from build123d import *

# Parameters (mm, degrees)
EXTRUDE_1_OUTLINE_W     = 2
EXTRUDE_1_OUTLINE_H     = 2
EXTRUDE_START           = -5
EXTRUDE_1_2_OUTLINE_R   = 4.25
EXTRUDE_1_2_OUTLINE_R_2 = 12
EXTRUDE_1_2_DEPTH       = 10
SKETCH_2_W              = 80
SKETCH_2_H              = 71
EXTRUDE_2_DEPTH         = 10
HOLE_START              = -6
HOLE_WIZARD_4_DEPTH     = 6.7
HOLE_START_2            = 0.7
HOLE_WIZARD_4_2_DEPTH   = 5.3
SKETCH_7_R              = 18
CUT_EXTRUDE_1_DEPTH     = 10
FILLET_2_R              = 5
FILLET_3_R              = 5
SKETCH_8_W              = 52.674698886
SKETCH_8_H              = 88.999999996
EXTRUDE_3_DEPTH         = 10
SKETCH_9_W              = 90.000000011
SKETCH_9_H              = 126.81088124
CUT_EXTRUDE_2_DEPTH     = 10
FILLET_4_R              = 10
FILLET_6_R              = 5


with BuildPart() as part:
    # 凸台-拉伸1: read off the stored shape, not the designer's step
    # 凸台-拉伸1 outline → 凸台-拉伸1 (revolve)
    with BuildSketch(Plane(origin=(0, -22.5, -28.5), x_dir=(0, 1, 0), z_dir=(0, 0, -1))):
        with Locations((11, -4)):
            Rectangle(EXTRUDE_1_OUTLINE_W, EXTRUDE_1_OUTLINE_H)
    revolve(axis=Axis((0, -22.5, -28.5), (1, 0, 0)))

    # Extrude 1 2 outline → Extrude 1 2 (add)
    with BuildSketch(Plane.YZ.offset(EXTRUDE_START)):
        with BuildLine():
            Line((114.999999996, 0), (-40, 0))
            ThreePointArc((-40, 0), (-43.535533906, -1.464466094), (-45, -5))
            Line((-45, -5), (-45, -148))
            Line((-45, -148), (-40, -153))
            Line((-40, -153), (-5, -153))
            Line((-5, -153), (1.7e-08, -147.999999983))
            Line((1.7e-08, -147.999999983), (0, -100))
            ThreePointArc((0, -100), (2.928932188, -92.928932188), (10, -90))
            Line((10, -90), (114.999999996, -90))
            Line((114.999999996, -90), (114.999999996, 0))
        make_face()
        with Locations((-22.5, -130.5)):
            Circle(EXTRUDE_1_2_OUTLINE_R, mode=Mode.SUBTRACT)
        with Locations((-22.5, -85.5)):
            Circle(EXTRUDE_1_2_OUTLINE_R, mode=Mode.SUBTRACT)
        with Locations((-22.5, -28.5)):
            Circle(EXTRUDE_1_2_OUTLINE_R_2, mode=Mode.SUBTRACT)
    extrude(amount=EXTRUDE_1_2_DEPTH)

    # Extrude 1 3 outline → Extrude 1 3 (revolve, cut)
    with BuildSketch(Plane(origin=(0, -22.5, -28.5), x_dir=(0, 1, 0), z_dir=(0, 0, -1))):
        Polygon((12, 5), (12, 4.5), (12.5, 5), align=None)
    revolve(axis=Axis((0, -22.5, -28.5), (1, 0, 0)), mode=Mode.SUBTRACT)

    # 草图2 → 凸台-拉伸2 (add)
    with BuildSketch(Plane.ZY.offset(5)):
        with Locations((40, 79.499999996)):
            Rectangle(SKETCH_2_W, SKETCH_2_H)
    extrude(amount=-EXTRUDE_2_DEPTH)

    # 打孔尺寸(%根据)内六角圆柱头螺钉的类型4: read off the stored shape, not the designer's step
    # 打孔尺寸(%根据)内六角圆柱头螺钉的类型4 outline → 打孔尺寸(%根据)内六角圆柱头螺钉的类型4 (cut)
    with BuildSketch(Plane.YZ.offset(HOLE_START)):
        with BuildLine():
            ThreePointArc((45.508621967, -3.732756057), (50.508621967, -8.732756057), (55.508621967, -3.732756057))
            Line((55.508621967, -3.732756057), (55.508621967, 15.767243943))
            ThreePointArc((55.508621967, 15.767243943), (50.508621967, 20.767243943), (45.508621967, 15.767243943))
            Line((45.508621967, 15.767243943), (45.508621967, -3.732756057))
        make_face()
        with BuildLine():
            ThreePointArc((55.508621967, 73.75), (50.508621967, 78.75), (45.508621967, 73.75))
            Line((45.508621967, 73.75), (45.508621967, 54.25))
            ThreePointArc((45.508621967, 54.25), (50.508621967, 49.25), (55.508621967, 54.25))
            Line((55.508621967, 54.25), (55.508621967, 73.75))
        make_face()
        with BuildLine():
            ThreePointArc((103.491378024, 54.25), (108.491378024, 49.25), (113.491378024, 54.25))
            Line((113.491378024, 54.25), (113.491378024, 73.75))
            ThreePointArc((113.491378024, 73.75), (108.491378024, 78.75), (103.491378024, 73.75))
            Line((103.491378024, 73.75), (103.491378024, 54.25))
        make_face()
        with BuildLine():
            ThreePointArc((113.491378024, 15.767243943), (108.491378024, 20.767243943), (103.491378024, 15.767243943))
            Line((103.491378024, 15.767243943), (103.491378024, -3.732756057))
            ThreePointArc((103.491378024, -3.732756057), (108.491378024, -8.732756057), (113.491378024, -3.732756057))
            Line((113.491378024, -3.732756057), (113.491378024, 15.767243943))
        make_face()
    extrude(amount=HOLE_WIZARD_4_DEPTH, mode=Mode.SUBTRACT)

    # Hole Wizard 4 2 outline → Hole Wizard 4 2 (cut)
    with BuildSketch(Plane.YZ.offset(HOLE_START_2)):
        with BuildLine():
            ThreePointArc((47.758621967, -3.732756057), (50.508621967, -6.482756057), (53.258621967, -3.732756057))
            Line((53.258621967, -3.732756057), (53.258621967, 15.767243943))
            ThreePointArc((53.258621967, 15.767243943), (50.508621967, 18.517243943), (47.758621967, 15.767243943))
            Line((47.758621967, 15.767243943), (47.758621967, -3.732756057))
        make_face()
        with BuildLine():
            ThreePointArc((53.258621967, 73.75), (50.508621967, 76.5), (47.758621967, 73.75))
            Line((47.758621967, 73.75), (47.758621967, 54.25))
            ThreePointArc((47.758621967, 54.25), (50.508621967, 51.5), (53.258621967, 54.25))
            Line((53.258621967, 54.25), (53.258621967, 73.75))
        make_face()
        with BuildLine():
            ThreePointArc((105.741378024, 54.25), (108.491378024, 51.5), (111.241378024, 54.25))
            Line((111.241378024, 54.25), (111.241378024, 73.75))
            ThreePointArc((111.241378024, 73.75), (108.491378024, 76.5), (105.741378024, 73.75))
            Line((105.741378024, 73.75), (105.741378024, 54.25))
        make_face()
        with BuildLine():
            ThreePointArc((111.241378024, 15.767243943), (108.491378024, 18.517243943), (105.741378024, 15.767243943))
            Line((105.741378024, 15.767243943), (105.741378024, -3.732756057))
            ThreePointArc((105.741378024, -3.732756057), (108.491378024, -6.482756057), (111.241378024, -3.732756057))
            Line((111.241378024, -3.732756057), (111.241378024, 15.767243943))
        make_face()
    extrude(amount=HOLE_WIZARD_4_2_DEPTH, mode=Mode.SUBTRACT)

    # 草图7 → 切除-拉伸1 (cut)
    with BuildSketch(Plane.ZY.offset(5)):
        with Locations((35.008621971, 64.999999996)):
            Circle(SKETCH_7_R)
    extrude(amount=-CUT_EXTRUDE_1_DEPTH, mode=Mode.SUBTRACT)

    # 圆角2
    fillet_2_edges = [part.edges().sort_by_distance(p)[0] for p in [
        (0, 114.999999996, -90),
        (0, 114.999999996, 80),
        (0, 43.999999996, 80),
    ]]
    fillet(fillet_2_edges, radius=FILLET_2_R)

    # 圆角3
    fillet_3_edges = [part.edges().sort_by_distance(p)[0] for p in [
        (0, 43.999999996, 0),
    ]]
    fillet(fillet_3_edges, radius=FILLET_3_R)

    # 草图8 → 凸台-拉伸3 (add)
    with BuildSketch(Plane.ZY.offset(5)):
        with Locations((18.662650557, -0.500000002)):
            Rectangle(SKETCH_8_W, SKETCH_8_H)
    extrude(amount=-EXTRUDE_3_DEPTH)

    # 草图9 → 切除-拉伸2 (cut)
    with BuildSketch(Plane.ZY.offset(5)):
        with Locations((-54.999999997, 63.40544062)):
            Rectangle(SKETCH_9_W, SKETCH_9_H)
    extrude(amount=-CUT_EXTRUDE_2_DEPTH, mode=Mode.SUBTRACT)

    # 圆角4
    fillet_4_edges = [part.edges().sort_by_distance(p)[0] for p in [
        (0, 43.999999996, 45),
        (0, 0, -9.999999991),
    ]]
    fillet(fillet_4_edges, radius=FILLET_4_R)

    # 圆角6
    fillet_6_edges = [part.edges().sort_by_distance(p)[0] for p in [
        (0, -45, 45),
        (0, 114.999999996, -9.999999991),
    ]]
    fillet(fillet_6_edges, radius=FILLET_6_R)


solid = part.part
Can you work these out from the model? Positions are in its coordinate system, mm. A direction names the side the tool comes from. Coordinates: 2 decimals unless noted, no trailing zeros. Write each loop counter-clockwise with the first axis right and the second up, starting at its lowest first coordinate (ties: lowest second). Pieces come first, ordered by that corner, then holes. Notation, with made-up numbers: (56, -39.75) - (67, -39.75) arc R8 ccw to (67, -34.75) - close; hole circle Ø5 at (57.5, 15). An arc over 180 degrees is marked (long way). Return JSON: item names as keys, results as strings. Group by question number.
Item 1: Please list where these lines run through material, in increasing order: probe 1 along Z at (x, y) = (-4.05, -22.5); probe 2 along Z at (x, y) = (0.5, -22.5); probe 3 along Y at (x, z) = (1.25, 58).
Item 2: If we section it at D-D (z = -28.5): Write out the boundary of the cut face in (x, y), then the cut area to 3 significant figures.
Item 3: I'm going to push flat-ended pins straight in: pin 1 Ø3 at (x, z) = (2, -53.5) entering from +Y; pin 2 Ø3 at (x, z) = (-2, 67) entering from -Y; pin 3 Ø5 at (y, z) = (110, 12) entering from -X; pin 4 Ø7 at (y, z) = (-22.5, -130.5) entering from -X. Where does each tip first touch, or does it pass through?
Item 4: Which directions (+Z, -Z, +X, -X, +Y, -Y) give clear straight access to the entire face, cutting with the end or side of a thin tool? Please do faces 4 (the face through (2.82, 50.448, -6.482)), 5 (the face through (-2, 103.491, 6)), 6 (the face through (0, -43, -150)).
Item 5: We'd pull the mould along Z, two halves only. Please class faces 1 (the face through (0.07, 41.15, 48.01)), 2 (the face through (2.82, 108.55, 76.5)), 3 (the face through (0, -45, -53)): pulls with the +Z half, pulls with the -Z half, needs draft (parallel to the pull), parting line crosses it, or undercut.
Item 6: If we section it at A-A (y = 65): Write out the boundary of the cut face in (x, z), then the cut area to 3 significant figures.
Item 7: If we section it at C-C (y = -22.5): Write out the boundary of the cut face in (x, z).
Item 8: If we section it at B-B (z = -85.5): Write out the boundary of the cut face in (x, y).
Return value:
{
 "1": {"probe 1": "z = -153 to -134.75, -126.25 to -89.75, -81.25 to -38.5, -18.5 to 45", "probe 2": "z = -153 to -134.75, -126.25 to -89.75, -81.25 to -40.5, -16.5 to 45", "probe 3": "y = 44 to 47.76, 53.26 to 105.74, 111.24 to 115"},
 "2": {"outline": "(-5, -45) - (5, -45) - (5, -35) - (4.5, -34.5) - (-3, -34.5) - (-3, -32.5) - (-5, -32.5) - close; (-5, -12.5) - (-3, -12.5) - (-3, -10.5) - (4.5, -10.5) - (5, -10) - (5, 0) - (-5, 0) - close", "area": "218 mm^2"},
 "3": {"pin 1": "stops at y = 0", "pin 2": "stops at y = 44", "pin 3": "stops at x = 0.7", "pin 4": "passes through"},
 "4": {"face 4": "+X, -X", "face 5": "-X", "face 6": "-Z, +X, -X, -Y"},
 "5": {"face 1": "pulls with the +Z half", "face 2": "undercut", "face 3": "needs draft"},
 "6": {"outline": "(-5, -10) - (5, -10) - (5, 17.01) - (-5, 17.01) - close; (-5, 53.01) - (5, 53.01) - (5, 80) - (-5, 80) - close", "area": "540 mm^2"},
 "7": {"outline": "(-5, -153) - (5, -153) - (5, -134.75) - (-5, -134.75) - close; (-5, -126.25) - (5, -126.25) - (5, -89.75) - (-5, -89.75) - close; (-5, -81.25) - (5, -81.25) - (5, -41) - (4.5, -40.5) - (-3, -40.5) - (-3, -38.5) - (-5, -38.5) - close; (-5, -18.5) - (-3, -18.5) - (-3, -16.5) - (4.5, -16.5) - (5, -16) - (5, 45) - (-5, 45) - close"},
 "8": {"outline": "(-5, -45) - (5, -45) - (5, -26.75) - (-5, -26.75) - close; (-5, -18.25) - (5, -18.25) - (5, 0) - (-5, 0) - close"}
}
